```python
from build123d import *

# Parameters (mm, degrees)
F0_W     = 70
F0_H     = 50
F1_DEPTH = 5
F2_W     = 4
F2_H     = 50
F3_DEPTH = 28
F4_R     = 5


with BuildPart() as f1:
    # F0 (on Top) → F1 (new body)
    with BuildSketch(Plane.XY):
        Rectangle(F0_W, F0_H)
    extrude(amount=F1_DEPTH)

    # F2 (on face) → F3 (join)
    with BuildSketch(Plane.XY.offset(5)):
        with Locations((-4.1, 0)):
            Rectangle(F2_W, F2_H)
        with Locations((4.1, 0)):
            Rectangle(F2_W, F2_H)
    extrude(amount=F3_DEPTH)

    # F4
    f4_edges = [f1.edges().sort_by_distance(p)[0] for p in [
        (-6.1, 0, 5),
        (6.1, 0, 5),
    ]]
    fillet(f4_edges, radius=F4_R)


solid = f1.part
```
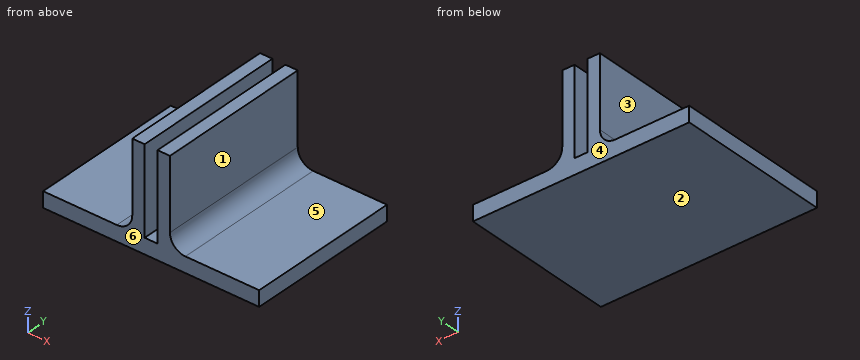
CAD build for the part. Positions are in the model's coordinates, mm. Face numbers are marked on the shaded views. A direction names the side the tool comes from. Coordinates: 2 decimals unless noted, no trailing zeros. Write each loop counter-clockwise with the first axis right and the second up, starting at its lowest first coordinate (ties: lowest second). Pieces come first, ordered by that corner, then holes. Notation, with made-up numbers: (88.25, 76.25) -> (137.25, 76.25) arc R37 ccw to (137.25, 115.25) -> close; hole circle Ø5 at (8, 76). An arc over 180 degrees is marked (long way). Return JSON: item names as keys, results as strings. Group by question number.
Q1. Which spindle directions (+Z, -Z, +X, -X, +Y, -Y) get a long thin tool onto all of the face, cutting with end or side? Do the marked faces 1, 2 and 3. Say none if no direction does.
Q2. Drill centre lines: line 1 (X direction, y = 10, z = 24); line 2 (Z direction, x = 26, y = 18.5); line 3 (X direction, y = 7.5, z = 8). Where is each one in solid material? Low to high.
Q3. Cut at A-A, the plane z = 21. Give the cut face in (x, y), then the cut area to 3 significant figures.
Q4. Flat gauge pins, fed straight in: pin 1 (1.5 mm diameter, centred on x = -24, y = 5, fed in from +Z); pin 2 (5 mm diameter, centred on y = 13, z = 17, fed in from +X); pin 3 (5 mm diameter, centred on y = -14, z = 28, fed in from -X). Where does each tip first touch, or does it go through?
Q5. Pull direction Y, two halves, no side cores. Call the marked faces 4, 5 and 6: released by +Y, released by -Y, zero draft, split by the parting line, or undercut.
Q6. Cut at C-C, the plane x = 28. Give the cut face in (y, z).
Q7. Cut at B-B, the plane y = 18. Give the cut face in (x, z).
Q8. Cut at D-D, the plane x = -10. Give the cut face in (y, z), then the cut area to 3 significant figures.
Returned:
{
 "1": {"face 1": "+Z, +X, +Y, -Y", "face 2": "-Z, +X, -X, +Y, -Y", "face 3": "+Z, -X, +Y, -Y"},
 "2": {"line 1": "x = -6.1 to -2.1, 2.1 to 6.1", "line 2": "z = 0 to 5", "line 3": "x = -6.52 to -2.1, 2.1 to 6.52"},
 "3": {"outline": "(-6.1, -25) -> (-2.1, -25) -> (-2.1, 25) -> (-6.1, 25) -> close; (2.1, -25) -> (6.1, -25) -> (6.1, 25) -> (2.1, 25) -> close", "area": "400 mm2"},
 "4": {"pin 1": "stops at z = 5", "pin 2": "stops at x = 6.1", "pin 3": "stops at x = -6.1"},
 "5": {"face 4": "released by +Y", "face 5": "zero draft", "face 6": "released by -Y"},
 "6": {"outline": "(-25, 0) -> (25, 0) -> (25, 5) -> (-25, 5) -> close"},
 "7": {"outline": "(-35, 0) -> (35, 0) -> (35, 5) -> (11.1, 5) arc R5 cw to (6.1, 10) -> (6.1, 33) -> (2.1, 33) -> (2.1, 5) -> (-2.1, 5) -> (-2.1, 33) -> (-6.1, 33) -> (-6.1, 10) arc R5 cw to (-11.1, 5) -> (-35, 5) -> close"},
 "8": {"outline": "(-25, 0) -> (25, 0) -> (25, 5.12) -> (-25, 5.12) -> close", "area": "256 mm2"}
}
